Verification items for the finished model (mm, model axes). A direction names the side the tool comes from. Give positions to 0.01 mm unless a question says otherwise; leave off trailing zeros. Write each loop counter-clockwise with the first axis right and the second up, starting at its lowest first coordinate (ties: lowest second). Pieces come first, ordered by that corner, then holes. Notation, with made-up numbers: (14.25, 17.25) -> (46.25, 17.25) arc R16 ccw to (46.25, 46.25) -> close; hole circle Ø7 at (-26.5, -36.5). An arc over 180 degrees is marked (long way). Answer as CSV lines item,"result".
```python
from build123d import *

# Parameters (mm, degrees)
SKETCH001_R      = 0.5
SKETCH001_W      = 18
SKETCH001_H      = 16
EXTRUDE001_DEPTH = 32
EXTRUDE_DEPTH    = 15


with BuildPart() as extrude001:
    # Sketch001 → Extrude001 (new body)
    with BuildSketch(Plane(origin=(0, 31, 0), x_dir=(-1, 0, 0), z_dir=(0, 1, 0))):
        with Locations((0, 7.5)):
            Circle(SKETCH001_R)
        with Locations((-17, -8)):
            Rectangle(SKETCH001_W, SKETCH001_H)
        with Locations((17, -8)):
            Rectangle(SKETCH001_W, SKETCH001_H)
    extrude(amount=-EXTRUDE001_DEPTH)


with BuildPart() as cut:
    # Sketch → Extrude (new body, symmetric)
    with BuildSketch(Plane.XY):
        Polygon((-13.5, 0), (-13.5, 29), (13.5, 29), (13.5, 0), (15, 0), (15, 30.5), (-15, 30.5), (-15, 0), align=None)
    extrude(amount=EXTRUDE_DEPTH, both=True)

    # Cut: cut Extrude001
    add(extrude001.part, mode=Mode.SUBTRACT)


solid = cut.part
```
1) Section check C-C (z = 7.5). Record the boundary of the cut face in (x, y), and give its area (4 significant figures).
Reported:
outline,"(-15, 0) -> (-13.5, 0) -> (-13.5, 29) -> (-0.5, 29) -> (-0.5, 30.5) -> (-15, 30.5) -> close; (0.5, 29) -> (13.5, 29) -> (13.5, 0) -> (15, 0) -> (15, 30.5) -> (0.5, 30.5) -> close"
area,"130.5 mm²"
2) Depth check by flat-ended pin: pin 1 (1.6 mm diameter, centred on y = 29.5, z = -6.5, fed in from +X); pin 2 (5.5 mm diameter, centred on x = 12, y = 8, fed in from -Z); pin 3 (0.8 mm diameter, centred on y = 29.5, z = -5, fed in from -X). Enter the tip coordinate at first touch or a pass-through.
Reported:
pin 1,"x = 8"
pin 2,"z = 0"
pin 3,"x = -8"
3) Section check A-A (y = 5). Record the boundary of the cut face in (x, z).
Reported:
outline,"(-15, 0) -> (-13.5, 0) -> (-13.5, 15) -> (-15, 15) -> close; (13.5, 0) -> (15, 0) -> (15, 15) -> (13.5, 15) -> close"
4) Draft check along X on faces 6 (the flat face through (14, 18, 0)), 7 (the flat face through (-15, 15, 8)), 8 (the flat face through (13.5, 15, 8)). Enter one of: +X half, -X half, draft (parallel to the pull), parting line (faces both ways), or undercut.
Reported:
face 6,"draft"
face 7,"-X half"
face 8,"undercut"
5) Section check D-D (x = -9.75). Record the boundary of the cut face in (y, z), and give its area (3 significant figures).
Reported:
outline,"(29, 0) -> (30.5, 0) -> (30.5, 15) -> (29, 15) -> close"
area,"22.5 mm²"
6) Section check B-B (x = 0). Record the boundary of the cut face in (y, z), and give its area (3 significant figures).
Reported:
outline,"(29, -15) -> (30.5, -15) -> (30.5, 7) -> (29, 7) -> close; (29, 8) -> (30.5, 8) -> (30.5, 15) -> (29, 15) -> close"
area,"43.5 mm²"
7) Tool access check on faces 1 (the flat face through (8, 30, -8)), 2 (the cylindrical face through (0, 30, 7)), 3 (the flat face through (-14, 18, 0)), 4 (the flat face through (-13.5, 14, 8)), 5 (the flat face through (0, 30.5, 4)). Record the directions out of +Z, -Z, +X, -X, +Y, -Y that give a thin tool (end or side, any length) a straight path to the whole face; none if there is none.
Reported:
face 1,"-Z, +X, +Y, -Y"
face 2,"+Y, -Y"
face 3,"-Z, -X, +Y, -Y"
face 4,"+Z, -Z, -Y"
face 5,"+Z, -Z, +X, -X, +Y"
8) Scan lines: line 1 along X through (y, z) = (17, 6.75); line 2 along Z through (x, y) = (0, 29.8); line 3 along Y through (x, z) = (-2.75, 0.25). Record each from-to range of solid material in increasing order.
Reported:
line 1,"-15 to -13.5, 13.5 to 15"
line 2,"-15 to 7, 8 to 15"
line 3,"29 to 30.5"
